from build123d import *

# Parameters (mm, degrees)
SKETCH1_W                                           = 101
SKETCH1_H                                           = 86.5
BOSS_EXTRUDE1_DEPTH                                 = 7
CBORE_FOR_M3_HEX_SOCKET_HEAD_CAP_SCREW1_D           = 3.4
CBORE_FOR_M3_HEX_SOCKET_HEAD_CAP_SCREW1_CBORE_D     = 6.5
CBORE_FOR_M3_HEX_SOCKET_HEAD_CAP_SCREW1_CBORE_DEPTH = 3.4
BOSS_EXTRUDE2_DEPTH                                 = 4
FILLET1_R                                           = 2
FILLET2_R                                           = 3
CUT_EXTRUDE2_DEPTH                                  = 68.392970702
CUT_EXTRUDE2_DEPTH_BACK                             = 68.392970702
SKETCH11_W                                          = 81
SKETCH11_H                                          = 37
SKETCH13_W                                          = 6
SKETCH13_H                                          = 6
SKETCH13_R                                          = 1.8
BOSS_EXTRUDE3_DEPTH                                 = 3
FILLET3_R                                           = 2


with BuildPart() as part:
    # Sketch1 → Boss-Extrude1 (new body)
    with BuildSketch(Plane(origin=(0, 0, 0), x_dir=(1, 0, 0), z_dir=(0, 1, 0))):
        Rectangle(SKETCH1_W, SKETCH1_H)
    extrude(amount=BOSS_EXTRUDE1_DEPTH)

    # CBORE for M3 Hex Socket Head Cap Screw1 (through all)
    with Locations(Plane(origin=(0, 7, 0), x_dir=(1, 0, 0), z_dir=(0, 1, 0))):
        with Locations((26.5, 39.25), (46.5, 19.25), (46.5, -19.25), (26.5, -39.25), (-26.5, -39.25), (-46.5, -19.25), (-46.5, 19.25), (-26.5, 39.25)):
            CounterBoreHole(CBORE_FOR_M3_HEX_SOCKET_HEAD_CAP_SCREW1_D / 2, CBORE_FOR_M3_HEX_SOCKET_HEAD_CAP_SCREW1_CBORE_D / 2, CBORE_FOR_M3_HEX_SOCKET_HEAD_CAP_SCREW1_CBORE_DEPTH)

    # Sketch8 → Boss-Extrude2 (add)
    with BuildSketch(Plane.XZ):
        Polygon((42, -34.75), (27, -34.75), (27, -29.75), (37, -29.75), (37, -19.75), (42, -19.75), align=None)
        Polygon((-42, -19.75), (-42, -34.75), (-27, -34.75), (-27, -29.75), (-37, -29.75), (-37, -19.75), align=None)
        Polygon((-42, 34.75), (-27, 34.75), (-27, 29.75), (-37, 29.75), (-37, 19.75), (-42, 19.75), align=None)
        Polygon((42, 19.75), (42, 34.75), (27, 34.75), (27, 29.75), (37, 29.75), (37, 19.75), align=None)
    extrude(amount=BOSS_EXTRUDE2_DEPTH)

    # Fillet1
    fillet1_edges = [part.edges().sort_by_distance(p)[0] for p in [
        (42, -2, 34.75),
        (27, -2, 34.75),
        (27, -2, 29.75),
        (37, -2, 29.75),
        (37, -2, 19.75),
        (42, -2, 19.75),
        (-42, -2, -34.75),
        (-27, -2, -34.75),
        (-27, -2, -29.75),
        (-37, -2, -29.75),
        (-37, -2, -19.75),
        (-42, -2, -19.75),
        (-37, -2, 19.75),
        (-37, -2, 29.75),
        (-27, -2, 29.75),
        (-27, -2, 34.75),
        (-42, -2, 34.75),
        (-42, -2, 19.75),
        (42, -2, -34.75),
        (42, -2, -19.75),
        (37, -2, -19.75),
        (37, -2, -29.75),
        (27, -2, -29.75),
        (27, -2, -34.75),
    ]]
    fillet(fillet1_edges, radius=FILLET1_R)

    # Fillet2
    fillet2_edges = [part.edges().sort_by_distance(p)[0] for p in [
        (50.5, 3.5, 43.25),
        (-50.5, 3.5, 43.25),
        (-50.5, 3.5, -43.25),
        (50.5, 3.5, -43.25),
    ]]
    fillet(fillet2_edges, radius=FILLET2_R)

    # Sketch11 → Cut-Extrude2 (cut, two sides: drawn at the far end of the back side and taken through both)
    with BuildSketch(Plane(origin=(0, 7, 0), x_dir=(1, 0, 0), z_dir=(0, 1, 0)).offset(-CUT_EXTRUDE2_DEPTH_BACK)):
        with Locations((0, -0.25)):
            Rectangle(SKETCH11_W, SKETCH11_H)
    extrude(amount=CUT_EXTRUDE2_DEPTH + CUT_EXTRUDE2_DEPTH_BACK, mode=Mode.SUBTRACT)

    # Sketch13 → Boss-Extrude3 (add)
    # profile 1 of 4: a face of its own
    with BuildSketch(Plane.XZ):
        with Locations((-37.5, 15.75)):
            Rectangle(SKETCH13_W, SKETCH13_H)
        with Locations(Location((-37.5, 15.75, 0), (0, 0, 90))):
            Circle(SKETCH13_R, mode=Mode.SUBTRACT)
    # profile 2 of 4: a face of its own
    with BuildSketch(Plane.XZ):
        with Locations((-37.5, -15.25)):
            Rectangle(SKETCH13_W, SKETCH13_H)
        with Locations(Location((-37.5, -15.25, 0), (0, 0, 270))):
            Circle(SKETCH13_R, mode=Mode.SUBTRACT)
    # profile 3 of 4: a face of its own
    with BuildSketch(Plane.XZ):
        with Locations((37.5, 15.75)):
            Rectangle(SKETCH13_W, SKETCH13_H)
        with Locations(Location((37.5, 15.75, 0), (0, 0, 270))):
            Circle(SKETCH13_R, mode=Mode.SUBTRACT)
    # profile 4 of 4: a face of its own
    with BuildSketch(Plane.XZ):
        with Locations((37.5, -15.25)):
            Rectangle(SKETCH13_W, SKETCH13_H)
        with Locations(Location((37.5, -15.25, 0), (0, 0, 90))):
            Circle(SKETCH13_R, mode=Mode.SUBTRACT)
    extrude(amount=-BOSS_EXTRUDE3_DEPTH)

    # Fillet3
    fillet3_edges = [part.edges().sort_by_distance(p)[0] for p in [
        (-40.5, 1.5, -12.25),
        (-34.5, 1.5, -12.25),
        (-34.5, 1.5, -18.25),
        (-34.5, 1.5, 18.75),
        (-34.5, 1.5, 12.75),
        (-40.5, 1.5, 12.75),
        (40.5, 1.5, 12.75),
        (34.5, 1.5, 12.75),
        (34.5, 1.5, 18.75),
        (34.5, 1.5, -18.25),
        (34.5, 1.5, -12.25),
        (40.5, 1.5, -12.25),
    ]]
    fillet(fillet3_edges, radius=FILLET3_R)


solid = part.part
Geometry check sheet. Reference: the model listing, model coordinates, mm. A direction names the side the tool comes from. Give positions to 0.01 mm unless a question says otherwise; leave off trailing zeros. Order: outer loops, then holes, each group sorted by start corner. A loop starts at its lowest first (then second) coordinate and runs counter-clockwise, first axis right, second up.
1. Depth check by flat-ended pin: pin 1 (1.2 mm diameter, centred on x = 34, y = -2, fed in from +Z); pin 2 (2 mm diameter, centred on x = 46.5, z = 18.5, fed in from +Y); pin 3 (4.5 mm diameter, centred on x = -37.5, z = -15.25, fed in from +Y). Enter the tip coordinate at first touch or a pass-through.
Completed:
pin 1: stops at z = 34.75
pin 2: stops at y = 3.6
pin 3: stops at y = 3
2. Draft check along Z on faces 4 (the face through (49.6, 3.55, -42.39)), 5 (the face through (-1, 0, -19)), 6 (the face through (42, -2, -27)). Enter one of: pulls with the +Z half, pulls with the -Z half, needs draft (parallel to the pull), parting line crosses it, or undercut.
Completed:
face 4: pulls with the -Z half
face 5: undercut
face 6: needs draft
3. Sectioned sample at B-B (z = 4.5). Record the boundary of the cut face in (x, y), then the cut area to 3 significant figures.
Completed:
outline: (-50.5, 0) - (-40.5, 0) - (-40.5, 7) - (-50.5, 7) - close; (40.5, 0) - (50.5, 0) - (50.5, 7) - (40.5, 7) - close
area: 140 mm2
4. Access from +Z, -Z, +X, -X, +Y, -Y to the whole of each face (thin tool, end or side, straight path). Record for faces 1 (the face through (-42, -2, 27)), 2 (the face through (-37, 3, -13)), 3 (the face through (37, -2, -25)).
Completed:
face 1: +Z, -Z, -X, -Y
face 2: +Y
face 3: -Y
5. Sectioned sample at A-A (x = -22). Record the boundary of the cut face in (y, z).
Completed:
outline: (0, -43.25) - (7, -43.25) - (7, -18.25) - (0, -18.25) - close; (0, 18.75) - (7, 18.75) - (7, 43.25) - (0, 43.25) - close
6. Sectioned sample at C-C (y = -2). State how many separate pieces and enclosed holes the cut face has, then the cut area to 3 significant figures.
Completed:
separate pieces: 4
enclosed holes: 0
area: 486 mm2
7. Scan lines: line 1 (X direction, y = 2.85, z = -39.25); line 2 (X direction, y = 1.35, z = 15.75); line 3 (Z direction, x = -26.5, y = 2.9). Record each from-to range of solid material in increasing order.
Completed:
line 1: x = -50.5 to -28.2, -24.8 to 24.8, 28.2 to 50.5
line 2: x = -50.5 to -39.3, -35.7 to -34.5, 34.5 to 35.7, 39.3 to 50.5
line 3: z = -43.25 to -40.95, -37.55 to -18.25, 18.75 to 37.55, 40.95 to 43.25
